Job drawing, mm, ordinate dimensions from the low corner. One solid piece. Coordinates: 2 decimals unless noted, no trailing zeros. Write each loop counter-clockwise with the first axis right and the second up, starting at its lowest first coordinate (ties: lowest second). Pieces come first, ordered by that corner, then holes. Notation, with made-up numbers: (-26, -6) -> (32, -6) arc R21 ccw to (32, 0) -> close; hole circle Ø9 at (-39, 35.5). An arc over 180 degrees is marked (long way). One line per question, with ' | ' between items. Start each with the question number.
Item 1: Saw through at A-A (z = 33.5). List the corners of the cut face in (x, y).
Item 2: Probe probe 1 along X at (y, z) = (1.3, 31); probe 2 along Z at (x, y) = (16, 3); probe 3 along Z at (x, y) = (28, 3.75) (1 decimal). List the from-to ranges inside material, lowest first. Write a range as [from, to].
Item 3: Saw through at D-D (z = 152). List the corners of the cut face in (x, y).
Item 4: Pin check, flat tips, straight feed: pin 1 (3 mm diameter, centred on x = 67.5, y = 3, fed in from +Z); pin 2 (1 mm diameter, centred on x = 34.5, y = 4.5, fed in from +Z); pin 3 (1.5 mm diameter, centred on x = 47, y = 1, fed in from +Z); pin 4 (1.5 mm diameter, centred on y = 2, z = 34.5, fed in from -X). Stop position of each tip, or through.
Item 5: Saw through at C-C (x = 119). List the corners of the cut face in (y, z).
Item 6: Saw through at B-B (y = 1.6). List the corners of the cut face in (x, z), and give its area (3 significant figures).
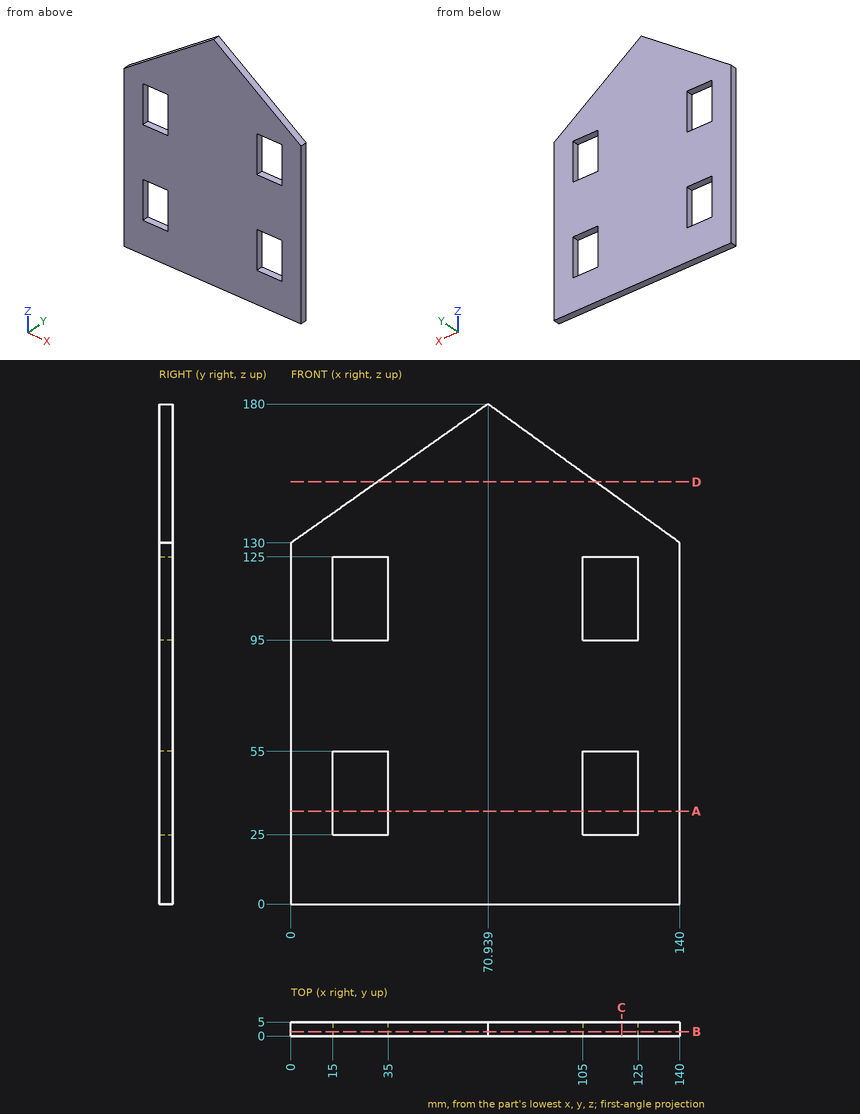
From the geometry:
1) outline: (0, 0) -> (15, 0) -> (15, 5) -> (0, 5) -> close; (35, 0) -> (105, 0) -> (105, 5) -> (35, 5) -> close; (125, 0) -> (140, 0) -> (140, 5) -> (125, 5) -> close
2) probe 1: [0, 15], [35, 105], [125, 140] | probe 2: [0, 25], [55, 95], [125, 141.28] | probe 3: [0, 25], [55, 95], [125, 149.7]
3) outline: (31.21, 0) -> (109.61, 0) -> (109.61, 5) -> (31.21, 5) -> close
4) pin 1: z = 178.63 | pin 2: z = 154.67 | pin 3: z = 163.66 | pin 4: x = 0
5) outline: (0, 0) -> (5, 0) -> (5, 25) -> (0, 25) -> close; (0, 55) -> (5, 55) -> (5, 95) -> (0, 95) -> close; (0, 125) -> (5, 125) -> (5, 145.2) -> (0, 145.2) -> close
6) outline: (0, 0) -> (140, 0) -> (140, 130) -> (70.94, 180) -> (0, 130) -> close; hole (15, 25) -> (35, 25) -> (35, 55) -> (15, 55) -> close; hole (15, 95) -> (35, 95) -> (35, 125) -> (15, 125) -> close; hole (105, 25) -> (125, 25) -> (125, 55) -> (105, 55) -> close; hole (105, 95) -> (125, 95) -> (125, 125) -> (105, 125) -> close | area: 19,300 mm2
